Here's how the part is built. I have some questions about the finished solid (model axes, mm). Face numbers are marked on the shaded views. A direction names the side the tool comes from. Round coordinates to 2 decimals unless told otherwise and drop trailing zeros. Write each loop counter-clockwise with the first axis right and the second up, starting at its lowest first coordinate (ties: lowest second). Pieces come first, ordered by that corner, then holes. Notation, with made-up numbers: (1, -0.5) -> (30, -0.5) arc R21 ccw to (30, 23.5) -> close; hole circle Ø2 at (87, -11). An arc over 180 degrees is marked (long way). Answer as CSV lines item,"result".
from build123d import *

# Parameters (mm, degrees)
SKETCH7_W           = 17.242861366
SKETCH7_H           = 40
BOSS_EXTRUDE1_DEPTH = 17.2
SKETCH8_W           = 29.242861366
SKETCH8_H           = 19.174682453
BOSS_EXTRUDE2_DEPTH = 5
SKETCH10_W          = 11.242861366
SKETCH10_H          = 11.2
CUT_EXTRUDE2_DEPTH  = 37
CUT_EXTRUDE3_REACH  = 43.972
SKETCH11_W          = 3
SKETCH11_H          = 16.077949268
FILLET1_R           = 1
SKETCH12_R          = 1.5
CUT_EXTRUDE4_DEPTH  = 5


with BuildPart() as part:
    # Sketch7 → Boss-Extrude1 (new body)
    with BuildSketch(Plane.XY):
        with Locations((0.869412251, 10.42274338)):
            Rectangle(SKETCH7_W, SKETCH7_H)
    extrude(amount=BOSS_EXTRUDE1_DEPTH)

    # Sketch8 → Boss-Extrude2 (add)
    with BuildSketch(Plane.XY):
        with Locations((0.869412251, 0.010084607)):
            Rectangle(SKETCH8_W, SKETCH8_H)
    extrude(amount=BOSS_EXTRUDE2_DEPTH)

    # Sketch10 → Cut-Extrude2 (cut)
    with BuildSketch(Plane(origin=(0, 30.42274338, 0), x_dir=(1, 0, 0), z_dir=(0, 1, 0))):
        with Locations((0.869412251, -8.6)):
            Rectangle(SKETCH10_W, SKETCH10_H)
    extrude(amount=-CUT_EXTRUDE2_DEPTH, mode=Mode.SUBTRACT)

    # Cut-Extrude3: up to this face of the body (flat: up to its plane)
    cut_extrude3_end = Plane(part.part.faces().sort_by_distance((9.490842934, 12.108695587, 9.587673627))[0])
    # Sketch11 → Cut-Extrude3 (cut, up to the picked face)
    with BuildSketch(Plane.ZY.offset(7.752018432), mode=Mode.PRIVATE) as cut_extrude3_sk1:
        with Locations((8.6, 10.42274338)):
            Rectangle(SKETCH11_W, SKETCH11_H)
    cut_extrude3_tool1 = split(extrude(cut_extrude3_sk1.sketch, amount=-CUT_EXTRUDE3_REACH, mode=Mode.PRIVATE), bisect_by=cut_extrude3_end, keep=Keep.BOTH, mode=Mode.PRIVATE)
    add(cut_extrude3_tool1.solids().sort_by(Axis((-7.752018, 10.422743, 8.6), (1, 0, 0)))[0], mode=Mode.SUBTRACT)

    # Fillet1
    fillet1_edges = [part.edges().sort_by_distance(p)[0] for p in [
        (7.990842934, 18.461718014, 10.1),
        (-6.252018432, 18.461718014, 10.1),
        (7.990842934, 2.383768746, 10.1),
        (-6.252018432, 2.383768746, 10.1),
        (7.990842934, 2.383768746, 7.1),
        (-6.252018432, 2.383768746, 7.1),
        (7.990842934, 18.461718014, 7.1),
        (-6.252018432, 18.461718014, 7.1),
    ]]
    fillet(fillet1_edges, radius=FILLET1_R)

    # Sketch12 → Cut-Extrude4 (cut)
    with BuildSketch(Plane.XY):
        with Locations((-10.752018432, 5.597425833)):
            Circle(SKETCH12_R)
        with Locations((-10.752018432, -6.411460604)):
            Circle(SKETCH12_R)
        with Locations(Location((12.490842934, -6.411460604, 0), (0, 0, 180))):
            Circle(SKETCH12_R)
        with Locations(Location((12.490842934, 5.597425833, 0), (0, 0, 180))):
            Circle(SKETCH12_R)
    extrude(amount=CUT_EXTRUDE4_DEPTH, mode=Mode.SUBTRACT)


solid = part.part
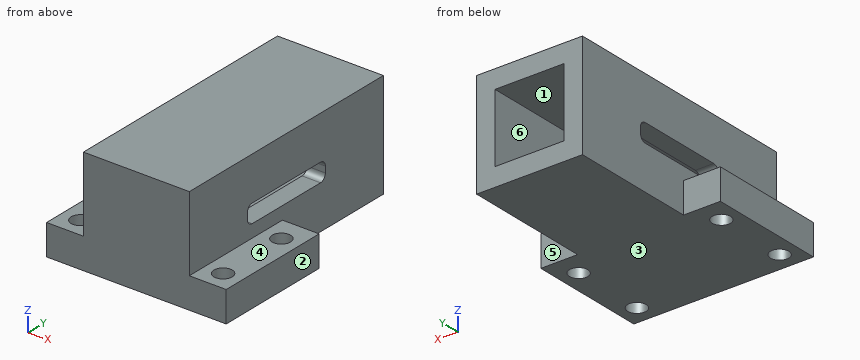
Item 1: For the marked faces 4, 5 and 6, which set-ups out of +Z, -Z, +X, -X, +Y, -Y let a thin tool reach every point of the face, with its end or its side?
Results found:
face 4,"+Z, +X, +Y, -Y"
face 5,"+Z, -Z, +X, +Y"
face 6,"+Y"
Item 2: Suppose I cut it at A-A, the plane y = 9. List the corners of the cut face in (x, z) for me.
Results found:
outline,"(-13.75, 0) -> (15.49, 0) -> (15.49, 5) -> (9.49, 5) -> (9.49, 7.1) -> (6.49, 7.1) -> (6.49, 3) -> (-4.75, 3) -> (-4.75, 7.1) -> (-7.75, 7.1) -> (-7.75, 5) -> (-13.75, 5) -> close; (-7.75, 10.1) -> (-4.75, 10.1) -> (-4.75, 14.2) -> (6.49, 14.2) -> (6.49, 10.1) -> (9.49, 10.1) -> (9.49, 17.2) -> (-7.75, 17.2) -> close"
Item 3: If we mould it in two halves opening along X, with no side actions, what happens to the marked faces 1, 2 and 3? For each: pulls with the +X half, pulls with the -X half, needs draft (parallel to the pull), parting line crosses it, or undercut.
Results found:
face 1,"undercut"
face 2,"pulls with the +X half"
face 3,"needs draft"
Item 4: I need wall thicknesses on L1, parallel to Z at x = 1.75, y = 12; L2, parallel to X at y = 5, z = 12.25; L3, parallel to Z at x = 9, y = 4. Which ranges of each line are inside material? Lowest first, please.
Results found:
L1,"z = 0 to 3, 14.2 to 17.2"
L2,"x = -7.75 to -4.75, 6.49 to 9.49"
L3,"z = 0 to 7.1, 10.1 to 17.2"
Item 5: Suppose I cut it at D-D, the plane z = 2. List the corners of the cut face in (x, y) for me, then the cut area to 3 significant figures.
Results found:
outline,"(-13.75, -9.58) -> (15.49, -9.58) -> (15.49, 9.6) -> (9.49, 9.6) -> (9.49, 30.42) -> (-7.75, 30.42) -> (-7.75, 9.6) -> (-13.75, 9.6) -> close; hole circle Ø3 at (-10.75, -6.41); hole circle Ø3 at (-10.75, 5.6); hole circle Ø3 at (12.49, -6.41); hole circle Ø3 at (12.49, 5.6)"
area,"892 mm²"
Item 6: Suppose I cut it at B-B, the plane y = -4. List the corners of the cut face in (x, z) for me, then the cut area to 3 significant figures.
Results found:
outline,"(-13.75, 0) -> (15.49, 0) -> (15.49, 5) -> (9.49, 5) -> (9.49, 17.2) -> (-7.75, 17.2) -> (-7.75, 5) -> (-13.75, 5) -> close; hole (-4.75, 3) -> (6.49, 3) -> (6.49, 14.2) -> (-4.75, 14.2) -> close"
area,"231 mm²"
Item 7: Will these pins go through, and if not, where does the flat tip stop? pin 1 (5 mm diameter, centred on x = 11.5, y = 1.5, fed in from +Z); pin 2 (9 mm diameter, centred on y = 20.5, z = 8, fed in from -X); pin 3 (8 mm diameter, centred on y = 21.5, z = 5, fed in from +X); pin 4 (1.8 mm diameter, centred on x = 12.49, y = -6.41, fed in from +Z).
Results found:
pin 1,"stops at z = 17.2"
pin 2,"stops at x = -7.75"
pin 3,"stops at x = 9.49"
pin 4,"passes through"
Item 8: Suppose I cut it at C-C, the plane x = 5. List the corners of the cut face in (y, z) for me, then the cut area to 3 significant figures.
Results found:
outline,"(-9.58, 0) -> (30.42, 0) -> (30.42, 3) -> (-6.58, 3) -> (-6.58, 14.2) -> (30.42, 14.2) -> (30.42, 17.2) -> (-9.58, 17.2) -> close"
area,"274 mm²"
